Verification items for the finished model (mm, model axes). Face numbers are marked on the shaded views. A direction names the side the tool comes from. Round coordinates to 2 decimals unless told otherwise and drop trailing zeros. Write each loop counter-clockwise with the first axis right and the second up, starting at its lowest first coordinate (ties: lowest second). Pieces come first, ordered by that corner, then holes. Notation, with made-up numbers: (-12, 73.5) - (46, 73.5) arc R30 cw to (46, 101.5) - close; hole circle Ø1 at (-37, 27.5). An arc over 180 degrees is marked (long way). Answer as a JSON object with one key per item and string values.
```python
from build123d import *

# Parameters (mm, degrees)
F1_DEPTH = 12.6
F2_W     = 6.2
F2_H     = 2
F3_DEPTH = 12.601
F2_W_2   = 3.5
F4_DEPTH = 12.601
F6_DEPTH = 12.701


with BuildPart() as f1:
    # F0 (on Front) → F1 (new body)
    with BuildSketch(Plane.XZ):
        Polygon((18.9, 0), (0, 0), (0, -10), (4.7, -10), (6.2, -12.6), (18.9, -12.6), align=None)
    extrude(amount=F1_DEPTH)

    # F2 (on face) → F3 (cut, through all)
    with BuildSketch(Plane(origin=(0, 0, -12.6), x_dir=(1, 0, 0), z_dir=(0, 0, -1))):
        with Locations((3.1, 6.3)):
            Rectangle(F2_W, F2_H)
    extrude(amount=-F3_DEPTH, mode=Mode.SUBTRACT)

    # F2 (on face) → F4 (cut, through all)
    with BuildSketch(Plane(origin=(0, 0, -12.6), x_dir=(1, 0, 0), z_dir=(0, 0, -1))):
        with Locations((17.15, 6.3)):
            Rectangle(F2_W_2, F2_H)
    extrude(amount=-F4_DEPTH, mode=Mode.SUBTRACT)

    # F5 (on face) → F6 (cut, through all)
    with BuildSketch(Plane(origin=(6.2, 0, 0), x_dir=(0, -1, 0), z_dir=(-1, 0, 0))):
        with BuildLine():
            ThreePointArc((5.3, -6.3), (6.3, -7.3), (7.3, -6.3))
            ThreePointArc((7.3, -6.3), (6.3, -5.3), (5.3, -6.3))
        make_face()
    extrude(amount=-F6_DEPTH, mode=Mode.SUBTRACT)


solid = f1.part
```
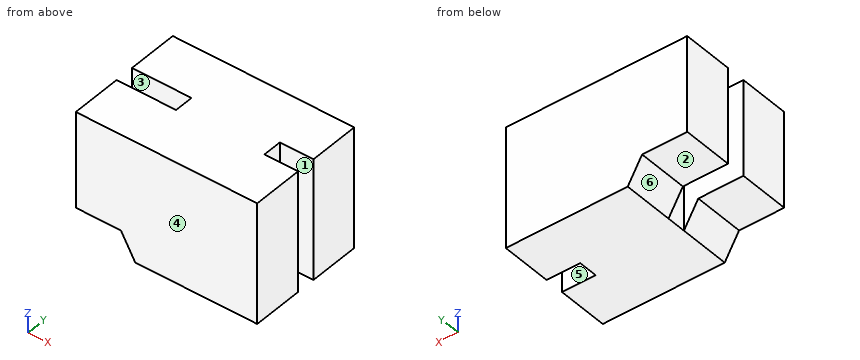
Q1. Section check D-D, the plane z = -6.75. Record the cut outline in (x, y), then the cut area to 3 significant figures.
Geometry check:
{"outline": "(0, -12.6) - (18.9, -12.6) - (18.9, -7.3) - (15.4, -7.3) - (15.4, -7.19) - (6.2, -7.19) - (6.2, -7.3) - (0, -7.3) - close; (0, -5.3) - (6.2, -5.3) - (6.2, -5.41) - (15.4, -5.41) - (15.4, -5.3) - (18.9, -5.3) - (18.9, 0) - (0, 0) - close", "area": "202 mm2"}
Q2. Set-up check for the marked faces 1, 2 and 3: record each of +Z, -Z, +X, -X, +Y, -Y from which the full face is reachable in a straight line by a thin tool's end or side.
Geometry check:
{"face 1": "+Z, -Z, +X", "face 2": "-Z, -X, +Y, -Y", "face 3": "+Z, -Z, -X"}
Q3. Material ranges on line 1 along Y through (x, z) = (9.5, -6.3); line 2 along Z through (x, y) = (2.25, -10.5), recorded low to high. Write a range as [from, to].
Geometry check:
{"line 1": "y = [-12.6, -7.3], [-5.3, 0]", "line 2": "z = [-10, 0]"}
Q4. Section check C-C, the plane z = -3.5. Record the cut outline in (x, y), then the cut area to 3 significant figures.
Geometry check:
{"outline": "(0, -12.6) - (18.9, -12.6) - (18.9, -7.3) - (15.4, -7.3) - (15.4, -5.3) - (18.9, -5.3) - (18.9, 0) - (0, 0) - (0, -5.3) - (6.2, -5.3) - (6.2, -7.3) - (0, -7.3) - close", "area": "219 mm2"}
Q5. Section check A-A, the plane y = -6.3. Record the cut outline in (x, z).
Geometry check:
{"outline": "(6.2, -12.6) - (15.4, -12.6) - (15.4, -7.3) - (6.2, -7.3) - close; (6.2, -5.3) - (15.4, -5.3) - (15.4, 0) - (6.2, 0) - close"}
Q6. Gauge pin test, flat ends, axial feed: P1, Ø6, axis at x = 6, z = -5.5, coming from the +Y side; P2, Ø0.6, axis at y = -6.5, z = -9, coming from the +X side; P3, Ø0.6, axis at y = -6, z = -8, coming from the -X side; P4, Ø5, axis at x = 1.5, y = -4, coming from the -Z side. Record the tip position at first contact, or that the pin passes through.
Geometry check:
{"P1": "stops at y = 0", "P2": "stops at x = 15.4", "P3": "stops at x = 6.2", "P4": "stops at z = -10"}
Q7. Release check for a two-part mould opening along Y. For the marked faces 4, 5 and 6 record: released by +Y, released by -Y, zero draft, split by the parting line, or undercut.
Geometry check:
{"face 4": "released by -Y", "face 5": "undercut", "face 6": "zero draft"}
Q8. Section check B-B, the plane x = 11.5. Record the cut outline in (y, z).
Geometry check:
{"outline": "(-12.6, -12.6) - (0, -12.6) - (0, 0) - (-12.6, 0) - close; hole circle Ø2 at (-6.3, -6.3)"}
